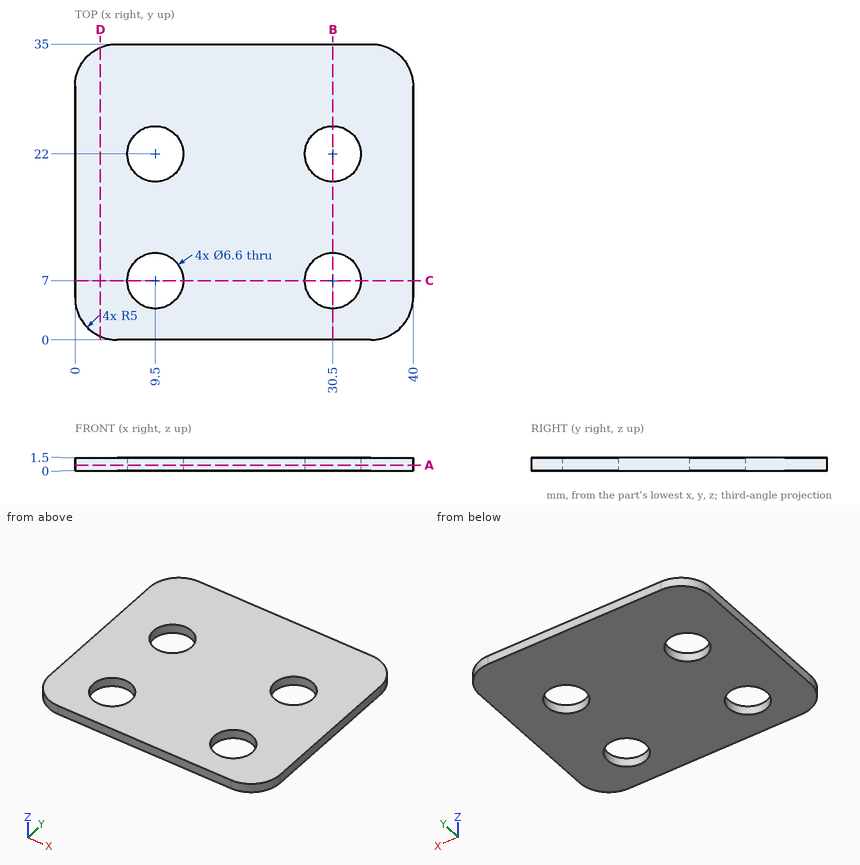
Geometry check sheet. Reference: drawing and pictorial views, mm from the part's lowest x, y, z. Give positions to 0.01 mm unless a question says otherwise; leave off trailing zeros. Order: outer loops, then holes, each group sorted by start corner. A loop starts at its lowest first (then second) coordinate and runs counter-clockwise, first axis right, second up. Notation, with made-up numbers: M -13.5,-5.5 L 37.5,-5.5 A19 ccw 37.5,8.5 Z; hole C -23.75,64 d6. An arc over 180 degrees is marked long. Answer in a Markdown table with one row per item.
1) Cross-section at B-B, the plane x = 30.5. Enter the section's corners in (y, z).
Filled sheet:
| item | result |
|---|---|
| outline | M 0,0 L 3.7,0 L 3.7,1.5 L 0,1.5 Z; M 10.3,0 L 18.7,0 L 18.7,1.5 L 10.3,1.5 Z; M 25.3,0 L 35,0 L 35,1.5 L 25.3,1.5 Z |
2) Cross-section at D-D, the plane x = 3. Enter the section's corners in (y, z).
Filled sheet:
| item | result |
|---|---|
| outline | M 0.42,0 L 34.58,0 L 34.58,1.5 L 0.42,1.5 Z |
3) Cross-section at A-A, the plane z = 0.65. Enter the section's corners in (x, y).
Filled sheet:
| item | result |
|---|---|
| outline | M 0,5 A5 ccw 5,0 L 35,0 A5 ccw 40,5 L 40,30 A5 ccw 35,35 L 5,35 A5 ccw 0,30 Z; hole C 9.5,7 d6.6; hole C 9.5,22 d6.6; hole C 30.5,7 d6.6; hole C 30.5,22 d6.6 |
4) Thickness scan on L1, parallel to Y at x = 30.5, z = 1.15; L2, parallel to X at y = 24.5, z = 0.9; L3, parallel to X at y = 8, z = 1.3. Record the ranges inside material, lowest first. Write a range as [from, to].
Filled sheet:
| item | result |
|---|---|
| L1 | y = [0, 3.7], [10.3, 18.7], [25.3, 35] |
| L2 | x = [0, 7.35], [11.65, 28.35], [32.65, 40] |
| L3 | x = [0, 6.36], [12.64, 27.36], [33.64, 40] |
5) Cross-section at C-C, the plane y = 7. Enter the section's corners in (x, z).
Filled sheet:
| item | result |
|---|---|
| outline | M 0,0 L 6.2,0 L 6.2,1.5 L 0,1.5 Z; M 12.8,0 L 27.2,0 L 27.2,1.5 L 12.8,1.5 Z; M 33.8,0 L 40,0 L 40,1.5 L 33.8,1.5 Z |
